Autodesk Inventor part; units mm, degrees
ref_plane "YZ Plane" through (0, 0, 0) normal (1, 0, 0) x (0, 1, 0)
ref_plane "XZ Plane" through (0, 0, 0) normal (0, 1, 0) x (-1, 0, 0)
ref_plane "XY Plane" through (0, 0, 0) normal (0, 0, 1) x (1, 0, 0)
sketch "Sketch1" plane through (0, 0, 0) normal (0, 1, 0) x (-1, 0, 0)
  line L0 (0, 0) -> (10, 0)
  line L1 (10, 0) -> (10, -20)
  line L2 (10, -20) -> (0, -20)
  line L3 (0, -20) -> (0, 0)
  dimension "d0" = 10
  dimension "d1" = 20
extrude "Extrusion1" add sketch "Sketch1" along normal blind 7
sketch "Sketch2" plane through (0, 7, 0) normal (0, 1, 0) x (1, 0, 0)
  line L0 (-10, 20) -> (-10, 0) construction
  line L1 (-5, 20) -> (-5, 0) construction
  line L2 (-10, 0) -> (0, 0) construction
  line L3 (-10, 10) -> (0, 10) construction
  line L4 (0, 0) -> (0, 20) construction
sketch "Sketch3" plane through (0, 7, 0) normal (0, 1, 0) x (1, 0, 0)
  point P0 (0, 0)
  point P1 (-5.1203, 3.6397)
hole "Hole1" at (-5.1203, 7, -3.6397) direction (0, -1, 0) diameter 2.85 depth 13.15 counterbore diameter 5.65 counterbore depth 3
sketch "Sketch4" plane through (0, 7, 0) normal (0, 1, 0) x (1, 0, 0)
  point P0 (0, 0)
  point P1 (-4.9804, 10.0094)
hole "Hole2" at (-4.9804, 7, -10.0094) direction (0, -1, 0) diameter 2.85 depth 9.05 counterbore diameter 5.65 counterbore depth 3
sketch "Sketch5" plane through (0, 7, 0) normal (0, 1, 0) x (1, 0, 0)
  point P0 (0, 0)
  point P1 (-8.0124, 17.6811)
hole "Hole3" at (-8.0124, 7, -17.6811) direction (0, -1, 0) diameter 3 end through all
sketch "Sketch6" plane through (0, 7, 0) normal (0, 1, 0) x (1, 0, 0)
  point P0 (0, 0)
  point P1 (-8.2667, 14.4)
hole "Hole4" at (-8.2667, 7, -14.4) direction (0, -1, 0) diameter 2 end through all
sketch "Sketch7" plane through (0, 7, 0) normal (0, 1, 0) x (1, 0, 0)
  point P0 (0, 0)
  point P1 (-4.5699, 15.3923)
hole "Hole5" at (-4.5699, 7, -15.3923) direction (0, -1, 0) diameter 4 end through all
sketch "Sketch8" plane through (0, 7, 0) normal (0, 1, 0) x (1, 0, 0)
  line L0 (0, 0) -> (0, 20)
  line L1 (0, 14.0043) -> (-1.4223, 12.582)
  line L2 (-1.4223, 12.582) -> (-1.4223, 19.3282)
  line L3 (-1.4223, 19.3282) -> (0, 17.9058)
  line L4 (0, 14.0043) -> (0, 17.9058)
  dimension "d39" = 45
  dimension "d40" = 45
  dimension "d41" = 6.7462
  dimension "d42" = 1.4223
extrude "Extrusion2" cut sketch "Sketch8" against normal through all
sketch "Sketch9" plane through (0, 7, 0) normal (0, 1, 0) x (1, 0, 0)
  line L0 (0, 14.0043) -> (0, 0)
  line L1 (0, 2.0269) -> (-1.0707, 0.9562)
  line L2 (-1.0707, 0.9562) -> (-1.0707, 6.9582)
  line L3 (-1.0707, 6.9582) -> (0, 5.8875)
  dimension "d45" = 45
  dimension "d46" = 45
  dimension "d47" = 6.002
  dimension "d48" = 1.0707
extrude "Extrusion3" cut sketch "Sketch9" against normal blind 7
equation "\"d40\" = d39"
equation "\"d46\" = d45"
properties part number "last_drill"
Read the model definition and answer for the solid it produces. Units are mm, in the model's axes. A direction names the side the tool comes from. Coordinates: 2 decimals unless noted, no trailing zeros. Loops run counter-clockwise (first coordinate to the right, second up) from the corner with the lowest first, then second, coordinate; pieces in that order, holes last. Notation, with made-up numbers: (85.25, -9.75) -> (130.25, -9.75) arc R24 cw to (130.25, 9.25) -> close; hole circle Ø10 at (-6, 70.25). An arc over 180 degrees is marked (long way). Write item = value, one per line. Start each with the question number.
1) The part is cut by section C-C, the plane z = -5.5. Determine the outline of the cut face in (x, y).
2) For faces 1 (the face through (-2.47, 5.48, -8.71)), 2 (the face through (-2.7, 7, -12.1)), 3 (the face through (-0.701, 3.549, -13.303)), determine the directions among +Z, -Z, +X, -X, +Y, -Y from which every point of the face is accessible in a straight line to the end or side of a thin tool.
3) The part is cut by section D-D, the plane z = -18.5. Determine the outline of the cut face in (x, y), plus the area to 3 significant figures.
4) Find the intervals of material crossed by L1, parallel to Z at x = -7.5, y = 1.25; L2, parallel to Z at x = -4, y = 5.5; L3, parallel to X at y = 6.25, z = -17.75, in increasing order. Write a range as from..to.
5) Given P1, Ø3, axis at x = -5.5, z = -4, coming from the +Y side, flat-ended and moving along its own axis, determine where the tip first touches the part or whether it passes through.
6) The part is cut by section A-A, the plane z = -14.25. Determine the outline of the cut face in (x, y), plus the area to 3 significant figures.
7) The part is cut by section B-B, the plane y = 1. State how many separate pieces and enclosed holes the cut face has, plus the area to 3 significant figures.
8) The mould has two halves that part along X. Classify faces 4 (the face through (-10, 3, -10)), 5 (the face through (-6, 4, -5)), 6 (the face through (-5, 3, 0)), 7 (the face through (0, 3, -10)): pulls with the +X half, pulls with the -X half, needs draft (parallel to the pull), parting line crosses it, or undercut.
Result:
q1.outline = (-10, 0) -> (-1.07, 0) -> (-1.07, 7) -> (-2.99, 7) -> (-2.99, 4) -> (-7.25, 4) -> (-7.25, 7) -> (-10, 7) -> close
q2.face_1 = +Y
q2.face_2 = +Z, -Z, +X, -X, +Y
q2.face_3 = +Y, -Y
q3.outline = (-10, 0) -> (-9.27, 0) -> (-9.27, 7) -> (-10, 7) -> close; (-6.76, 0) -> (-1.42, 0) -> (-1.42, 7) -> (-6.76, 7) -> close; (-0.59, 0) -> (0, 0) -> (0, 7) -> (-0.59, 7) -> close
q3.area = 46.6 mm²
q4.L1 = -20..-19.09, -16.27..-15.04, -13.76..0
q4.L2 = -20..-17.31, -13.48..-12.66, -7.36..-6.23, -1.05..0
q4.L3 = -10..-9.51, -6.51..-1.42
q5.P1 = 4
q6.outline = (-10, 0) -> (-9.26, 0) -> (-9.26, 7) -> (-10, 7) -> close; (-7.28, 0) -> (-6.21, 0) -> (-6.21, 7) -> (-7.28, 7) -> close; (-2.93, 0) -> (-1.42, 0) -> (-1.42, 7) -> (-2.93, 7) -> close
q6.area = 23.2 mm²
q7.separate_pieces = 1
q7.enclosed_holes = 5
q7.area = 152 mm²
q8.face_4 = pulls with the -X half
q8.face_5 = undercut
q8.face_6 = needs draft
q8.face_7 = pulls with the +X half
